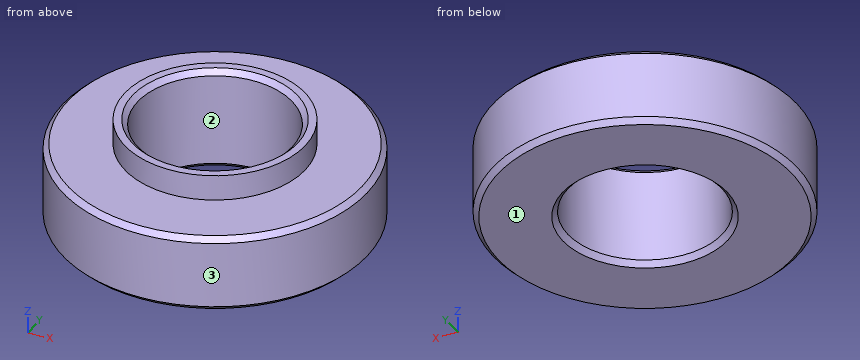
from build123d import *

# Parameters (mm, degrees)
F0_R     = 5.9
F1_DEPTH = 3
F2_R     = 3.5
F3_DEPTH = 1
F4_R     = 3
F5_DEPTH = 4.001
F6_SIZE  = 0.2


with BuildPart() as f1:
    # F0 (on Top) → F1 (new body)
    with BuildSketch(Plane.XY):
        Circle(F0_R)
    extrude(amount=F1_DEPTH)

    # F2 (on face) → F3 (join)
    with BuildSketch(Plane.XY.offset(3)):
        Circle(F2_R)
    extrude(amount=F3_DEPTH)

    # F4 (on face) → F5 (cut, through all)
    with BuildSketch(Plane(origin=(0, 0, 0), x_dir=(1, 0, 0), z_dir=(0, 0, -1))):
        Circle(F4_R)
    extrude(amount=-F5_DEPTH, mode=Mode.SUBTRACT)

    # F6
    f6_edges = [f1.edges().sort_by_distance(p)[0] for p in [
        (-5.9, 0, 3),
        (-5.9, 0, 0),
        (-3, 0, 0),
        (-3, 0, 4),
    ]]
    chamfer(f6_edges, length=F6_SIZE)


solid = f1.part
Could you check a few things on this model? Use its own coordinates, in mm. Face numbers are marked on the shaded views. Round coordinates to 2 decimals unless told otherwise and drop trailing zeros. Loops run counter-clockwise (first coordinate to the right, second up) from the corner with the lowest first, then second, coordinate; pieces in that order, holes last. Notation, with made-up numbers: (54, 40.5) - (93, 40.5) arc R23 ccw to (93, 78.5) - close; hole circle Ø9 at (12.5, 36.25). An arc over 180 degrees is marked (long way). Write item = value, one per line.
1) I'm going to push a flat-ended pin straight in: P1, Ø1.5, axis at y = 4.5, z = 1.5, coming from the -X side. Where does the tip first touch, or does it pass through?
Computed:
P1 = -4.55
2) Imagine slicing it at D-D (z = 3.5). Please give me the cut outline in (x, y), and give its area (3 significant figures).
Computed:
outline = circle Ø7 at (0, 0); hole circle Ø6 at (0, 0)
area = 10.2 mm2
3) Imagine slicing it at A-A (y = 0). Please give me the cut outline in (x, z), and give its area (3 significant figures).
Computed:
outline = (-5.9, 0.2) - (-5.7, 0) - (-3.2, 0) - (-3, 0.2) - (-3, 3.8) - (-3.2, 4) - (-3.5, 4) - (-3.5, 3) - (-5.7, 3) - (-5.9, 2.8) - close; (3, 0.2) - (3.2, 0) - (5.7, 0) - (5.9, 0.2) - (5.9, 2.8) - (5.7, 3) - (3.5, 3) - (3.5, 4) - (3.2, 4) - (3, 3.8) - close
area = 18.2 mm2
4) Imagine slicing it at C-C (z = 1.9). Please give me the cut outline in (x, y).
Computed:
outline = circle Ø11.8 at (0, 0); hole circle Ø6 at (0, 0)
5) If we mould it in two halves opening along X, with no side actions, what happens to the marked faces 1, 2 and 3? For each: pulls with the +X half, pulls with the -X half, needs draft (parallel to the pull), parting line crosses it, or undercut.
Computed:
face_1 = needs draft
face_2 = undercut
face_3 = parting line crosses it
6) I need wall thicknesses on line 1 along Y through (x, z) = (0, 2.6); line 2 along Z through (x, y) = (5.25, 0.5); line 3 along Y through (x, z) = (-2.5, 0.75). Which ranges of each line are inside material? Lowest first, please. Write a range as from..to.
Computed:
line_1 = -5.9..-3, 3..5.9
line_2 = 0..3
line_3 = -5.34..-1.66, 1.66..5.34
